Geometry: final body of the model. Coordinates: model frame, mm. Coordinates: 2 decimals unless noted, no trailing zeros. Order: outer loops, then holes, each group sorted by start corner. A loop starts at its lowest first (then second) coordinate and runs counter-clockwise, first axis right, second up. Notation, with made-up numbers: M -31.75,59 L -19.75,59 A33 cw -19.75,96 Z; hole C 9,2 d6. An arc over 180 degrees is marked long. Write item = value, one per line. Start each with the question number.
Autodesk Inventor part; units mm, degrees
ref_plane "YZ Plane" through (0, 0, 0) normal (1, 0, 0) x (0, 1, 0)
ref_plane "XZ Plane" through (0, 0, 0) normal (0, 1, 0) x (-1, 0, 0)
ref_plane "XY Plane" through (0, 0, 0) normal (0, 0, 1) x (1, 0, 0)
sketch "Sketch2" plane through (0, 0, 0) normal (0, 0, 1) x (1, 0, 0)
  circle A0 centre (0, 0) radius 62.5
  circle A1 centre (0, 0) radius 110
  dimension "d25" = 125
  dimension "d27" = 220
extrude "Plate2" add sketch "Sketch2" along normal blind 8
sketch "Sketch3" plane through (0, 0, 8) normal (0, 0, 1) x (1, 0, 0)
  circle A0 centre (-90, 0) radius 8.5
  circle A1 centre (0, 0) radius 90 construction
  dimension "d28" = 180
  dimension "d15" = 17
extrude "Cut1" cut sketch "Sketch3" against normal blind 8
pattern_circular "Circular Pattern1" count 4 over 360 about axis through (0, 0, -10) along (0, 0, 1) of "Cut1"
equation "\"d17\" = Thickness"
equation "\"d14\" = Thickness"
equation "\"BendReliefWidth\" = Thickness"
equation "\"BendReliefDepth\" = 0.5 * Thickness"
equation "\"CornerReliefSize\" = 4 * Thickness"
equation "\"MinimumRemnant\" = 2 * Thickness"
equation "\"TransitionRadius\" = BendRadius"
equation "\"JacobiRadiusSize\" = BendRadius"
equation "\"GapSize\" = Thickness"
properties part number "APN 1431 FDS flange DN90" material "Steel"
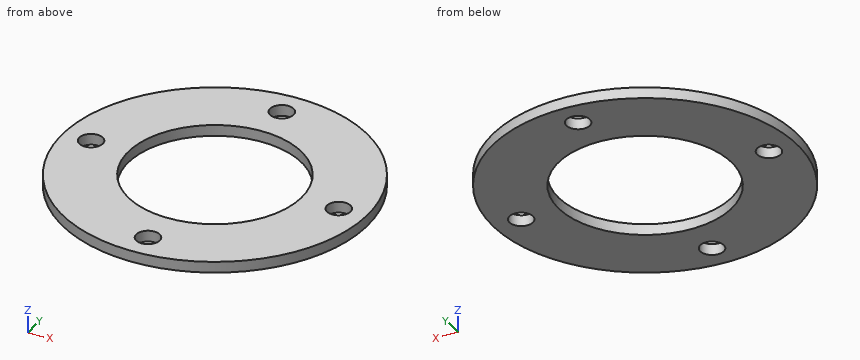
Item 1: Section query A-A on y = -92. Output: boundary loops of the cut face in (x, z).
Item 2: Section query C-C on x = 45. Output: boundary loops of the cut face in (y, z), and give its area (3 significant figures).
Item 3: Material intervals for probe 1 along X at (y, z) = (-6.5, 3.25); probe 2 along Y at (x, z) = (92.5, 6.75); probe 3 along X at (y, z) = (-87, 2.25), sorted ascending. Write a range as [from, to].
Item 4: Section query B-B on z = 6. Output: boundary loops of the cut face in (x, y).
Item 5: Section query D-D on y = 0. Output: boundary loops of the cut face in (x, z).
Item 6: First-contact query: pin 1 (4 mm diameter, centred on y = -70.5, z = 6.5, fed in from +X); pin 2 (4 mm diameter, centred on x = 82.5, z = 1.5, fed in from -Y) (3 decimals); pin 3 (3 mm diameter, centred on y = -46, z = 6, fed in from +X). Flat tips, straight axial feed; report the tip coordinate or a pass-through.
Ans:
q1.outline = M -60.3,0 L -8.26,0 L -8.26,8 L -60.3,8 Z; M 8.26,0 L 60.3,0 L 60.3,8 L 8.26,8 Z
q2.outline = M -100.37,0 L -43.37,0 L -43.37,8 L -100.37,8 Z; M 43.37,0 L 100.37,0 L 100.37,8 L 43.37,8 Z
q2.area = 912 mm^2
q3.probe_1 = [-109.81, -95.48], [-84.52, -62.16], [62.16, 84.52], [95.48, 109.81]
q3.probe_2 = [-59.53, -8.12], [8.12, 59.53]
q3.probe_3 = [-67.31, -7.95], [7.95, 67.31]
q4.outline = C 0,0 d220; hole C -90,0 d17; hole C 0,0 d125; hole C 0,-90 d17; hole C 0,90 d17; hole C 90,0 d17
q5.outline = M -110,0 L -98.5,0 L -98.5,8 L -110,8 Z; M -81.5,0 L -62.5,0 L -62.5,8 L -81.5,8 Z; M 62.5,0 L 81.5,0 L 81.5,8 L 62.5,8 Z; M 98.5,0 L 110,0 L 110,8 L 98.5,8 Z
q6.pin_1 = 86.07
q6.pin_2 = -74.965
q6.pin_3 = 100.6
